Work out the finished part from the listing and answer in its coordinate system (mm). A direction names the side the tool comes from. Round coordinates to 2 decimals unless told otherwise and drop trailing zeros. Write each loop counter-clockwise with the first axis right and the second up, starting at its lowest first coordinate (ties: lowest second). Pieces come first, ordered by that corner, then holes.
1. Determine the mould class of faces 4 (the face through (0, 0, -12)), 5 (the face through (-25.715, 1.014, -30.899)), 6 (the face through (16.199, 0.986, -22.915)) for opening direction X: pulls with the +X half, pulls with the -X half, needs draft (parallel to the pull), parting line crosses it, or undercut.
2. Find section C-C (z = -21.5). Write down the section's boundary in (x, y).
3. Find section B-B (z = -8). Write down the section's boundary in (x, y), and give its area (3 significant figures).
4. Flat-ended cylindrical pins translate along their axes: pin 1 Ø1.2 at (x, y) = (-24, 1.5) entering from +Z (3 decimals); pin 2 Ø4 at (x, z) = (-17, -17) entering from -Y; pin 3 Ø2.5 at (x, z) = (-22.5, -27.7) entering from +Y; pin 4 Ø1 at (x, y) = (18, 1) entering from +Z. Find the tip coordinate at first contact, or state that the pin passes through.
5. Find section D-D (y = 0.9). Count the separate pieces of the cut face and the enclosed holes in it, and give its area (3 significant figures).
6. A tool of negligible diameter and unlimited length cuts with its end or side. For faces 1 (the face through (24, 1, -24.2)), 2 (the face through (16.5, 1, -18)), 3 (the face through (-24, 1, -24.2)), from which of +Z, -Z, +X, -X, +Y, -Y can it reach the whole face along a straight path? Write none if from no direction.
7. Find section A-A (x = -17.5). Write down the section's boundary in (y, z).
8. Straight lines are drawn through the part: probe 1 along X at (y, z) = (0.75, -8); probe 2 along Z at (x, y) = (-0.5, 1.7); probe 3 along X at (y, z) = (1.2, -17). For each, find the intervals that lie inside material, in ascending order.
```python
from build123d import *

# Parameters (mm, degrees)
SKETCH_1_R          = 1.5
EXTRUDE_1_DEPTH     = 2
SKETCH_2_R          = 1
SKETCH_2_W          = 33
SKETCH_2_H          = 10.2
CUT_EXTRUDE_1_DEPTH = 41.662513449
FILLET_1_R          = 1


with BuildPart() as part:
    # 草图1 → 凸台-拉伸1 (new body)
    with BuildSketch(Plane(origin=(0, 0, 0), x_dir=(1, 0, 0), z_dir=(0, 1, 0))):
        Polygon((-22.5, 3), (-22.5, 24.2), (-26, 24.2), (-26, 31.2), (26, 31.2), (26, 24.2), (22.5, 24.2), (22.5, 3), (12.5, 3), (12.5, 0), (-12.5, 0), (-12.5, 3), align=None)
        with Locations(Location((-22.5, 27.7, 0), (0, 0, 270))):
            Circle(SKETCH_1_R, mode=Mode.SUBTRACT)
        with Locations(Location((22.5, 27.7, 0), (0, 0, 90))):
            Circle(SKETCH_1_R, mode=Mode.SUBTRACT)
        with Locations(Location((-17.5, 8, 0), (0, 0, 270))):
            Circle(SKETCH_1_R, mode=Mode.SUBTRACT)
        with Locations(Location((17.5, 8, 0), (0, 0, 90))):
            Circle(SKETCH_1_R, mode=Mode.SUBTRACT)
    extrude(amount=EXTRUDE_1_DEPTH)

    # 草图2 → 切除-拉伸1 (cut, through all)
    with BuildSketch(Plane(origin=(0, 2, 0), x_dir=(1, 0, 0), z_dir=(0, 1, 0))):
        with Locations((-13.5, 3)):
            Circle(SKETCH_2_R)
        with Locations((13.5, 3)):
            Circle(SKETCH_2_R)
        with Locations((0, 18.1)):
            Rectangle(SKETCH_2_W, SKETCH_2_H)
    extrude(amount=-CUT_EXTRUDE_1_DEPTH, mode=Mode.SUBTRACT)

    # 圆角1
    fillet_1_edges = [part.edges().sort_by_distance(p)[0] for p in [
        (26, 1, -24.2),
        (22.5, 1, -24.2),
        (22.5, 1, -3),
        (12.5, 1, 0),
        (-12.5, 1, 0),
        (-22.5, 1, -3),
        (-22.5, 1, -24.2),
        (-26, 1, -24.2),
        (-26, 1, -31.2),
        (26, 1, -31.2),
        (-16.5, 1, -13),
        (-16.5, 1, -23.2),
        (16.5, 1, -23.2),
        (16.5, 1, -13),
    ]]
    fillet(fillet_1_edges, radius=FILLET_1_R)


solid = part.part
```
Worked answers:
1. face 4: needs draft
1. face 5: pulls with the -X half
1. face 6: undercut
2. outline: (-22.5, 0) - (-16.5, 0) - (-16.5, 2) - (-22.5, 2) - close; (16.5, 0) - (22.5, 0) - (22.5, 2) - (16.5, 2) - close
3. outline: (-22.5, 0) - (-19, 0) - (-19, 2) - (-22.5, 2) - close; (-16, 0) - (16, 0) - (16, 2) - (-16, 2) - close; (19, 0) - (22.5, 0) - (22.5, 2) - (19, 2) - close
3. area: 78.0 mm2
4. pin 1: stops at z = -24.195
4. pin 2: stops at y = 0
4. pin 3: passes through
4. pin 4: stops at z = -3
5. separate pieces: 1
5. enclosed holes: 5
5. area: 1,020 mm2
6. face 1: +Z, +X, +Y, -Y
6. face 2: +Y, -Y
6. face 3: +Z, -X, +Y, -Y
7. outline: (0, -31.2) - (2, -31.2) - (2, -9.5) - (0, -9.5) - close; (0, -6.5) - (2, -6.5) - (2, -3) - (0, -3) - close
8. probe 1: x = -22.5 to -19, -16 to 16, 19 to 22.5
8. probe 2: z = -31.2 to -23.2, -13 to 0
8. probe 3: x = -22.5 to -16.5, 16.5 to 22.5
